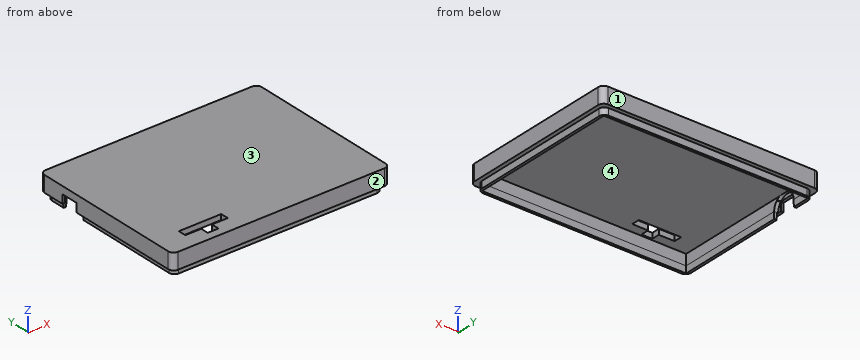
```python
from build123d import *

# Parameters (mm, degrees)
ESQUISSE1_W              = 81
ESQUISSE1_H              = 61
ESQUISSE1_W_2            = 76
ESQUISSE1_H_2            = 56
EXTRU_MINCE1_DEPTH       = 6
EXTRU_MINCE2_OUTLINE_W   = 77.912724676
EXTRU_MINCE2_OUTLINE_H   = 57.912724676
EXTRU_MINCE2_OUTLINE_W_2 = 76.087275324
EXTRU_MINCE2_OUTLINE_H_2 = 56.087275324
EXTRU_MINCE2_DEPTH       = 2.5
EXTRU_MINCE2_DRAFT       = -1
ESQUISSE3_W              = 76
ESQUISSE3_H              = 56
BOSS_EXTRU_1_DEPTH       = 2
CONG_1_R                 = 2
CONG_2_R                 = 2
ESQUISSE4_W              = 10
ESQUISSE4_H              = 6.5
ENL_V_MAT_EXTRU_1_DEPTH  = 12
ENL_V_MAT_EXTRU_2_DEPTH  = 1.5
ENL_V_MAT_EXTRU_3_DEPTH  = 11.5


# Read off the part's stored shape, not the designer's step: Extru.-Mince2
with BuildPart() as part:
    # Esquisse1 → Extru.-Mince1 (new body)
    with BuildSketch(Plane.XY):
        with Locations((40.5, 30.5)):
            Rectangle(ESQUISSE1_W, ESQUISSE1_H)
        with Locations((40.5, 30.5)):
            Rectangle(ESQUISSE1_W_2, ESQUISSE1_H_2, mode=Mode.SUBTRACT)
    extrude(amount=EXTRU_MINCE1_DEPTH)


with BuildPart() as extru_mince2_tool:
    # Extru.-Mince2 outline → Extru.-Mince2 (with draft: the straight prism first)
    with BuildSketch(Plane.XY.offset(-2.5)):
        with Locations((40.5, 30.5)):
            Rectangle(EXTRU_MINCE2_OUTLINE_W, EXTRU_MINCE2_OUTLINE_H)
        with Locations((40.5, 30.5)):
            Rectangle(EXTRU_MINCE2_OUTLINE_W_2, EXTRU_MINCE2_OUTLINE_H_2, mode=Mode.SUBTRACT)
    extrude(amount=EXTRU_MINCE2_DEPTH)
    # Extru.-Mince2: the draft: its side faces are tilted about the plane it starts from
    extru_mince2_sides = [extru_mince2_tool.faces().sort_by_distance(p)[0] for p in [
        (1.543637662, 30.5, -1.25),
        (40.5, 1.543637662, -1.25),
        (79.456362338, 30.5, -1.25),
        (40.5, 59.456362338, -1.25),
        (40.5, 2.456362338, -1.25),
        (2.456362338, 30.5, -1.25),
        (40.5, 58.543637662, -1.25),
        (78.543637662, 30.5, -1.25),
    ]]
    draft(extru_mince2_sides, Plane.XY.offset(-2.5), EXTRU_MINCE2_DRAFT)


with BuildPart() as part_1:
    add(part.part)

    # Extru.-Mince2: add extru_mince2_tool
    add(extru_mince2_tool.part)

    # Esquisse3 → Boss.-Extru.1 (add)
    with BuildSketch(Plane.XY.offset(6)):
        with Locations((40.5, 30.5)):
            Rectangle(ESQUISSE3_W, ESQUISSE3_H)
    extrude(amount=-BOSS_EXTRU_1_DEPTH)

    # Cong_1
    cong_1_edges = [part_1.edges().sort_by_distance(p)[0] for p in [
        (1.521818831, 59.478181169, -1.25),
        (79.478181169, 59.478181169, -1.25),
        (79.478181169, 1.521818831, -1.25),
        (1.521818831, 1.521818831, -1.25),
    ]]
    fillet(cong_1_edges, radius=CONG_1_R)

    # Cong_2
    cong_2_edges = [part_1.edges().sort_by_distance(p)[0] for p in [
        (0, 61, 3),
        (81, 61, 3),
        (81, 0, 3),
        (0, 0, 3),
    ]]
    fillet(cong_2_edges, radius=CONG_2_R)

    # Esquisse4 → Enl_v. mat.-Extru.1 (cut)
    with BuildSketch(Plane(origin=(0, 0, 0), x_dir=(0, 0, -1), z_dir=(1, 0, 0))):
        with Locations((1.75, 47.55)):
            Rectangle(ESQUISSE4_W, ESQUISSE4_H)
    extrude(amount=ENL_V_MAT_EXTRU_1_DEPTH, mode=Mode.SUBTRACT)

    # Esquisse5 → Enl_v. mat.-Extru.2 (cut)
    with BuildSketch(Plane(origin=(2.499238534, 0, -0.043624371), x_dir=(-0.01745240643728355, 0, -0.9998476951563913), z_dir=(0.9998476951563913, 0, -0.01745240643728355))):
        with BuildLine():
            Line((-0.043631016, 52.05), (9.11559923, 52.05))
            Line((9.11559923, 52.05), (9.11559923, 43.05))
            Line((9.11559923, 43.05), (-0.043631016, 43.05))
            ThreePointArc((-0.043631016, 43.05), (-4.543631016, 47.55), (-0.043631016, 52.05))
        make_face()
    extrude(amount=-ENL_V_MAT_EXTRU_2_DEPTH, mode=Mode.SUBTRACT)

    # Esquisse6 → Enl_v. mat.-Extru.3 (cut)
    with BuildSketch(Plane.XY):
        Polygon((25.54, 9.14), (9.74, 9.14), (9.74, 6.14), (15.64, 6.14), (15.64, 3.14), (19.64, 3.14), (19.64, 6.14), (25.54, 6.14), align=None)
    extrude(amount=ENL_V_MAT_EXTRU_3_DEPTH, mode=Mode.SUBTRACT)


solid = part_1.part
```
Input: part model. Units: mm. Frame: model coordinates. Face numbers are marked on the shaded views. Coordinates: 2 decimals unless noted, no trailing zeros. Write each loop counter-clockwise with the first axis right and the second up, starting at its lowest first coordinate (ties: lowest second). Pieces come first, ordered by that corner, then holes.
1) Material intervals for line 1 along X through (y, z) = (55, 2.5); line 2 along Y through (x, z) = (35.5, 0.5); line 3 along Y through (x, z) = (63, -1.5), sorted ascending.
2) Section B-B on y = 20. Output: boundary loops of the cut face in (x, z).
3) Pin query (flat end, axial travel): pin 1 Ø12 at (x, y) = (41.5, 41.5) entering from -Z; pin 2 Ø0.5 at (x, z) = (1.5, -1) entering from +Y; pin 3 Ø0.8 at (x, z) = (2, -1.5) entering from -Y. Return the tip coordinate at first contact, or that it passes through.
4) Section C-C on x = 27. Output: boundary loops of the cut face in (y, z).
5) Mould query, pull axis Y, two halves, no side actions, for the marked faces 1, 2, 3 and 4. Classes: pulls with the +Y half, pulls with the -Y half, needs draft (parallel to the pull), parting line crosses it, or undercut.
6) Section A-A on x = 18. Output: boundary loops of the cut face in (y, z), and give its area (3 significant figures).
Check result:
1. line 1: x = 0 to 2.5, 78.5 to 81
1. line 2: y = 0 to 2.5, 58.5 to 61
1. line 3: y = 1.53 to 2.47, 58.53 to 59.47
2. outline: (0, 0) - (1.5, 0) - (1.54, -2.5) - (2.46, -2.5) - (2.5, 0) - (2.5, 4) - (78.5, 4) - (78.5, 0) - (78.54, -2.5) - (79.46, -2.5) - (79.5, 0) - (81, 0) - (81, 6) - (0, 6) - close
3. pin 1: stops at z = 4
3. pin 2: stops at y = 58.42
3. pin 3: stops at y = 1.87
4. outline: (0, 0) - (1.5, 0) - (1.54, -2.5) - (2.46, -2.5) - (2.5, 0) - (2.5, 4) - (58.5, 4) - (58.5, 0) - (58.54, -2.5) - (59.46, -2.5) - (59.5, 0) - (61, 0) - (61, 6) - (0, 6) - close
5. face 1: pulls with the +Y half
5. face 2: pulls with the -Y half
5. face 3: needs draft
5. face 4: undercut
6. outline: (0, 0) - (1.5, 0) - (1.54, -2.5) - (2.46, -2.5) - (2.5, 0) - (2.5, 4) - (3.14, 4) - (3.14, 6) - (0, 6) - close; (9.14, 4) - (58.5, 4) - (58.5, 0) - (58.54, -2.5) - (59.46, -2.5) - (59.5, 0) - (61, 0) - (61, 6) - (9.14, 6) - close
6. area: 135 mm2
